```python
from build123d import *

# Parameters (mm, degrees)
F0_W     = 475
F0_H     = 2282
F1_DEPTH = 18
F2_W     = 40
F2_H     = 20
F3_DEPTH = 2282


with BuildPart() as f1:
    # F0 (on Front) → F1 (new body)
    with BuildSketch(Plane.XZ):
        with Locations((237.5, 1141)):
            Rectangle(F0_W, F0_H)
    extrude(amount=F1_DEPTH)

    # F2 (on face) → F3 (join)
    with BuildSketch(Plane(origin=(0, 0, 0), x_dir=(1, 0, 0), z_dir=(0, 0, -1))):
        with Locations((20, 28)):
            Rectangle(F2_W, F2_H)
        with Locations((455, 28)):
            Rectangle(F2_W, F2_H)
    extrude(amount=-F3_DEPTH)


solid = f1.part
```
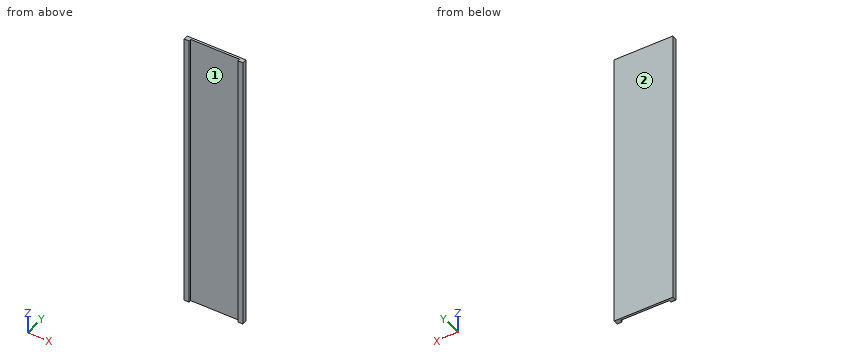
Here's how the part is built. I have some questions about the finished solid (model axes, mm). Face numbers are marked on the shaded views. Round coordinates to 2 decimals unless told otherwise and drop trailing zeros. Order: outer loops, then holes, each group sorted by start corner. A loop starts at its lowest first (then second) coordinate and runs counter-clockwise, first axis right, second up. Notation, with made-up numbers: M -11,-6 L 14,-6 A16 ccw 14,1 Z; hole C 13,-5 d1. An arc over 180 degrees is marked long. Answer as CSV lines item,"result".
Item 1: Imagine slicing it at C-C on x = 157. List the corners of the cut face in (y, z) for me, and give its area (3 significant figures).
From the geometry:
outline,"M -18,0 L 0,0 L 0,2282 L -18,2282 Z"
area,"41,100 mm2"
Item 2: We'd pull the mould along X, two halves only. Please class the marked faces 1 and 2: +X half, -X half, draft (parallel to the pull), parting line (faces both ways), or undercut.
From the geometry:
face 1,"undercut"
face 2,"draft"
Item 3: Imagine slicing it at A-A on y = -26. List the corners of the cut face in (x, z) for me, and give its area (3 significant figures).
From the geometry:
outline,"M 0,0 L 40,0 L 40,2282 L 0,2282 Z; M 435,0 L 475,0 L 475,2282 L 435,2282 Z"
area,"183,000 mm2"
Item 4: Please list where these lines run through material, in increasing order: L1, parallel to X at y = -34, z = 252.5; L2, parallel to Y at x = 308, z = 296. Write a range as [from, to].
From the geometry:
L1,"[0, 40], [435, 475]"
L2,"[-18, 0]"
Item 5: Imagine slicing it at B-B on z = 1088. List the corners of the cut face in (x, y) for me.
From the geometry:
outline,"M 0,-38 L 40,-38 L 40,-18 L 435,-18 L 435,-38 L 475,-38 L 475,0 L 0,0 Z"
